```python
from build123d import *

# Parameters (mm, degrees)
EXTRUDE_1_DEPTH     = 10
SKETCH_2_W          = 10
SKETCH_2_H          = 10
SKETCH_2_W_2        = 6.15
SKETCH_2_H_2        = 6.15
EXTRUDE_2_DEPTH     = 10
EXTRUDE_START       = 10
SKETCH_2_3_W        = 6.15
SKETCH_2_3_H        = 6.15
EXTRUDE_3_DEPTH     = 50
CUT_EXTRUDE_1_DEPTH = 87.372217755
SKETCH_4_R          = 1.65
CUT_EXTRUDE_2_DEPTH = 77.00668145
FILLET_1_R          = 1


with BuildPart() as part:
    # 草图1 → 凸台-拉伸1 (new body)
    with BuildSketch(Plane.XY):
        Polygon((0, 18.8), (0, -18.8), (40, -18.8), (40, -24.8), (-10, -24.8), (-10, 24.8), (40, 24.8), (40, 18.8), align=None)
    extrude(amount=EXTRUDE_1_DEPTH)

    # 草图2 → 凸台-拉伸2 (add)
    # profile 1 of 2: a face of its own
    with BuildSketch(Plane.ZY.offset(10)):
        with Locations((5, 0)):
            Rectangle(SKETCH_2_W, SKETCH_2_H)
        with Locations((5, 0)):
            Rectangle(SKETCH_2_W_2, SKETCH_2_H_2, mode=Mode.SUBTRACT)
    # profile 2 of 2: a face of its own
    with BuildSketch(Plane.ZY.offset(10)):
        with Locations((5, 0)):
            Rectangle(SKETCH_2_W_2, SKETCH_2_H_2)
    extrude(amount=EXTRUDE_2_DEPTH)

    # 草图2<3> → 凸台-拉伸3 (add)
    with BuildSketch(Plane.ZY.offset(10).offset(EXTRUDE_START)):
        with Locations((5, 0)):
            Rectangle(SKETCH_2_3_W, SKETCH_2_3_H)
    extrude(amount=EXTRUDE_3_DEPTH)

    # 草图3 → 切除-拉伸1 (cut, through all)
    with BuildSketch(Plane(origin=(0, 24.8, 0), x_dir=(1, 0, 0), z_dir=(0, 1, 0))):
        with BuildLine():
            ThreePointArc((32.35, -5), (35, -7.65), (37.65, -5))
            Line((37.65, -5), (32.35, -5))
        make_face()
        with BuildLine():
            Line((32.35, -5), (37.65, -5))
            ThreePointArc((37.65, -5), (35, -2.35), (32.35, -5))
        make_face()
        with BuildLine():
            ThreePointArc((35, 0), (38.535533906, -1.464466094), (40, -5))
            Line((40, -5), (40, 0))
            Line((40, 0), (35, 0))
        make_face()
        with BuildLine():
            Line((40, -10), (40, -5))
            ThreePointArc((40, -5), (38.535533906, -8.535533906), (35, -10))
            Line((35, -10), (40, -10))
        make_face()
    extrude(amount=-CUT_EXTRUDE_1_DEPTH, mode=Mode.SUBTRACT)

    # 草图4 → 切除-拉伸2 (cut, through all)
    with BuildSketch(Plane(origin=(0, 3.075, 0), x_dir=(1, 0, 0), z_dir=(0, 1, 0))):
        with Locations(Location((-45, -5, 0), (0, 0, 180))):
            Circle(SKETCH_4_R)
        with Locations(Location((-32.5, -5, 0), (0, 0, 180))):
            Circle(SKETCH_4_R)
        with Locations(Location((-57.5, -5, 0), (0, 0, 180))):
            Circle(SKETCH_4_R)
    extrude(amount=-CUT_EXTRUDE_2_DEPTH, mode=Mode.SUBTRACT)

    # 圆角1
    fillet_1_edges = [part.edges().sort_by_distance(p)[0] for p in [
        (-45, -3.075, 1.925),
        (-45, -3.075, 8.075),
        (-45, 3.075, 8.075),
        (-45, 3.075, 1.925),
    ]]
    fillet(fillet_1_edges, radius=FILLET_1_R)


solid = part.part
```
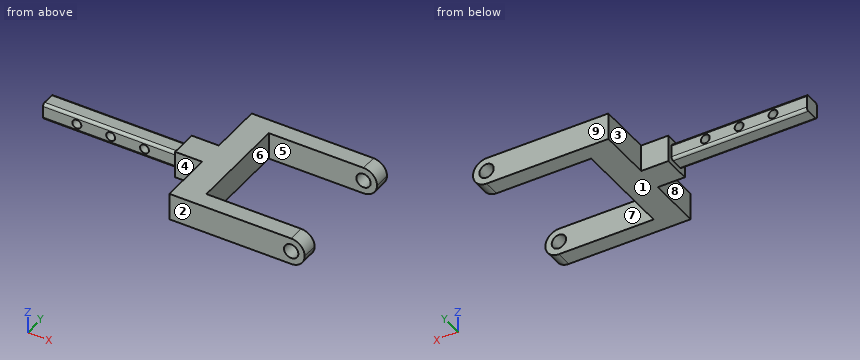
Geometry check sheet. Reference: the model listing, model coordinates, mm. Face numbers are marked on the shaded views. A direction names the side the tool comes from. Round coordinates to 2 decimals unless told otherwise and drop trailing zeros. Loops run counter-clockwise (first coordinate to the right, second up) from the corner with the lowest first, then second, coordinate; pieces in that order, holes last. Notation, with made-up numbers: M -23,-14 L 27,-14 A35 ccw 27,24 Z; hole C 89.5,25 d1. An arc over 180 degrees is marked long. Return JSON: item names as keys, results as strings. Group by question number.
(1) Section check C-C, the plane y = -15. Enter the section's corners in (x, z).
(2) Set-up check for the marked faces 1, 2, 3, 4 and 5: record each of +Z, -Z, +X, -X, +Y, -Y from which the full face is reachable in a straight line by a thin tool's end or side.
(3) Mould release check, pull along Y, two halves, no side actions. Record for the marked faces 6, 7, 8 and 9: pulls with the +Y half, pulls with the -Y half, needs draft (parallel to the pull), parting line crosses it, or undercut.
(4) Section check D-D, the plane x = 21. Enter the section's corners in (y, z), and give its area (3 significant figures).
(5) Section check A-A, the plane x = -57.5. Enter the section's corners in (y, z) (3 decimals).
(6) Scan lines: line 1 along Z through (x, y) = (35, 21.35); line 2 along Y through (x, z) = (8, 3.5); line 3 along X through (y, z) = (-22.3, 5). Record each from-to range of solid material in increasing order. Write a range as [from, to].
(7) Section check B-B, the plane x = -23.5. Enter the section's corners in (y, z) (3 decimals), and give its area (3 significant figures).
(8) Go/stop test with flat-tipped pins: pin 1 (4 mm diameter, centred on y = 9.5, z = 2, fed in from -X); pin 2 (4.5 mm diameter, centred on x = -45, z = 6, fed in from +Y) (3 decimals); pin 3 (3 mm diameter, centred on x = -17, z = 4.5, fed in from +Y). Record where each tip stops, or that it passes through.
Data:
{
 "1": {"outline": "M -10,0 L 0,0 L 0,10 L -10,10 Z"},
 "2": {"face 1": "-Z, +X, -X, +Y, -Y", "face 2": "+Z, -Z, +X, -X, -Y", "face 3": "+Z, -Z, -X, +Y", "face 4": "+Z, -Z, -X, -Y", "face 5": "+Z, -Z, +X"},
 "3": {"face 6": "undercut", "face 7": "undercut", "face 8": "needs draft", "face 9": "pulls with the +Y half"},
 "4": {"outline": "M -24.8,0 L -18.8,0 L -18.8,10 L -24.8,10 Z; M 18.8,0 L 24.8,0 L 24.8,10 L 18.8,10 Z", "area": "120 mm²"},
 "5": {"outline": "M -3.075,2.925 A1 ccw -2.075,1.925 L 2.075,1.925 A1 ccw 3.075,2.925 L 3.075,3.35 L -3.075,3.35 Z; M -3.075,6.65 L 3.075,6.65 L 3.075,7.075 A1 ccw 2.075,8.075 L -2.075,8.075 A1 ccw -3.075,7.075 Z"},
 "6": {"line 1": "[0, 2.35], [7.65, 10]", "line 2": "[-24.8, -18.8], [18.8, 24.8]", "line 3": "[-10, 32.35], [37.65, 40]"},
 "7": {"outline": "M -3.075,2.925 A1 ccw -2.075,1.925 L 2.075,1.925 A1 ccw 3.075,2.925 L 3.075,7.075 A1 ccw 2.075,8.075 L -2.075,8.075 A1 ccw -3.075,7.075 Z", "area": "37.0 mm²"},
 "8": {"pin 1": "x = -10", "pin 2": "y = 3.075", "pin 3": "y = 5"}
}
